```python
from build123d import *

# Parameters (mm, degrees)
SKETCH1_R           = 8.89
BOSS_EXTRUDE2_DEPTH = 9.525
SKETCH1_7_R         = 8.89
BOSS_EXTRUDE4_DEPTH = 22.225


with BuildPart() as part:
    # Sketch1 → Boss-Extrude2 (new body)
    # profile 1 of 5: a face of its own
    with BuildSketch(Plane(origin=(0, 0, 0), x_dir=(0, 0, -1), z_dir=(1, 0, 0))):
        with BuildLine():
            add(Edge.make_bspline(
                [(14.974900338, 11.775179823), (12.331090746, 14.230118369), (9.525, 16.497783942)],
                knots=[1.475431476, 1.475431476, 1.475431476, 1.652003752, 1.652003752, 1.652003752], degree=2, weights=[0.938489801, 0.965564284, 1]))
            ThreePointArc((9.525, 16.497783942), (4.930502809, 18.400886991), (0, 19.05))
            ThreePointArc((0, 19.05), (-10.677275343, 15.776510744), (-17.68505503, 7.0810542))
            add(Edge.make_bspline(
                [(-17.68505503, 7.0810542), (-18.489189379, 3.563978658), (-19.05, 0)],
                knots=[4.617024129, 4.617024129, 4.617024129, 4.793596405, 4.793596405, 4.793596405], degree=2, weights=[0.938489801, 0.965564284, 1]))
            ThreePointArc((-19.05, 0), (-18.400886991, -4.930502809), (-16.497783942, -9.525))
            ThreePointArc((-16.497783942, -9.525), (-8.324221416, -17.135047062), (2.710154692, -18.856234023))
            add(Edge.make_bspline(
                [(2.710154692, -18.856234023), (6.158098634, -17.794097027), (9.525, -16.497783942)],
                knots=[1.475431476, 1.475431476, 1.475431476, 1.652003752, 1.652003752, 1.652003752], degree=2, weights=[0.938489801, 0.965564284, 1]))
            ThreePointArc((9.525, -16.497783942), (13.470384182, -13.470384182), (16.497783942, -9.525))
            ThreePointArc((16.497783942, -9.525), (18.400886991, -4.930502809), (19.05, 0))
            ThreePointArc((19.05, 0), (18.002421385, 6.230194562), (14.974900338, 11.775179823))
        make_face()
        Circle(SKETCH1_R, mode=Mode.SUBTRACT)
    # profile 2 of 5: a face of its own
    with BuildSketch(Plane(origin=(0, 0, 0), x_dir=(0, 0, -1), z_dir=(1, 0, 0))):
        Circle(SKETCH1_R)
        Polygon((2.822954141, -4.8895), (5.645908282, 0), (2.822954141, 4.8895), (-2.822954141, 4.8895), (-5.645908282, 0), (-2.822954141, -4.8895), align=None, mode=Mode.SUBTRACT)
    # profile 3 of 5: a face of its own
    with BuildSketch(Plane(origin=(0, 0, 0), x_dir=(0, 0, -1), z_dir=(1, 0, 0))):
        with BuildLine():
            ThreePointArc((-17.68505503, 7.0810542), (-10.677275343, 15.776510744), (0, 19.05))
            ThreePointArc((0, 19.05), (2.161493982, 32.047813076), (8.413309173, 43.646520237))
            add(Edge.make_bspline(
                [(8.413309173, 43.646520237), (-8.576070469, 46.921395365), (-17.68505503, 7.0810542)],
                knots=[3.141592654, 3.141592654, 3.141592654, 4.617024129, 4.617024129, 4.617024129], degree=2, weights=[1, 0.712256416, 0.938489801]))
        make_face()
    # profile 4 of 5: a face of its own
    with BuildSketch(Plane(origin=(0, 0, 0), x_dir=(0, 0, -1), z_dir=(1, 0, 0))):
        with BuildLine():
            ThreePointArc((-16.497783942, -9.525), (-28.83496725, -14.151997839), (-42.005649898, -14.537120645))
            add(Edge.make_bspline(
                [(-42.005649898, -14.537120645), (-36.347085133, -30.887792574), (2.710154692, -18.856234023)],
                knots=[0, 0, 0, 1.475431476, 1.475431476, 1.475431476], degree=2, weights=[1, 0.712256416, 0.938489801]))
            ThreePointArc((2.710154692, -18.856234023), (-8.324221416, -17.135047062), (-16.497783942, -9.525))
        make_face()
    # profile 5 of 5: a face of its own
    with BuildSketch(Plane(origin=(0, 0, 0), x_dir=(0, 0, -1), z_dir=(1, 0, 0))):
        with BuildLine():
            add(Edge.make_bspline(
                [(33.592340725, -29.109399592), (44.923155602, -16.033602792), (14.974900338, 11.775179823)],
                knots=[0, 0, 0, 1.475431476, 1.475431476, 1.475431476], degree=2, weights=[1, 0.712256416, 0.938489801]))
            ThreePointArc((14.974900338, 11.775179823), (18.002421385, 6.230194562), (19.05, 0))
            ThreePointArc((19.05, 0), (18.400886991, -4.930502809), (16.497783942, -9.525))
            ThreePointArc((16.497783942, -9.525), (26.673473268, -17.895815237), (33.592340725, -29.109399592))
        make_face()
    extrude(amount=BOSS_EXTRUDE2_DEPTH)

    # Sketch1_7 → Boss-Extrude4 (add)
    with BuildSketch(Plane(origin=(0, 0, 0), x_dir=(0, 0, -1), z_dir=(1, 0, 0))):
        Circle(SKETCH1_7_R)
        Polygon((2.822954141, -4.8895), (5.645908282, 0), (2.822954141, 4.8895), (-2.822954141, 4.8895), (-5.645908282, 0), (-2.822954141, -4.8895), align=None, mode=Mode.SUBTRACT)
    extrude(amount=BOSS_EXTRUDE4_DEPTH)


solid = part.part
```
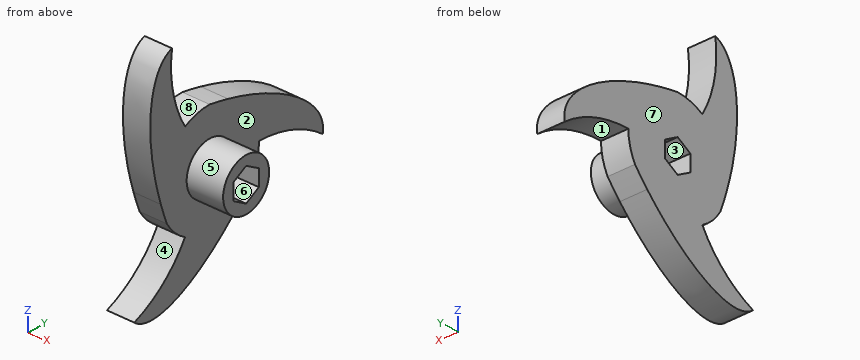
Verification items for the finished model (mm, model axes). Face numbers are marked on the shaded views. A direction names the side the tool comes from. Give positions to 0.01 mm unless a question says otherwise; leave off trailing zeros. Order: outer loops, then holes, each group sorted by start corner. A loop starts at its lowest first (then second) coordinate and runs counter-clockwise, first axis right, second up. Notation, with made-up numbers: M 79.25,54 L 120.25,54 A18 cw 120.25,64 Z; hole C 35,-21.75 d2. An arc over 180 degrees is marked long. Answer in a Markdown table with one row per item. Add a question column.
Item 1: Mould release check, pull along Y, two halves, no side actions. Record for the marked faces 5, 6, 7 and 8: released by +Y, released by -Y, zero draft, split by the parting line, or undercut.
Item 2: Tool access check on the marked faces 1, 2, 3 and 4. Record the directions out of +Z, -Z, +X, -X, +Y, -Y that give a thin tool (end or side, any length) a straight path to the whole face; none if there is none.
Item 3: Gauge pin test, flat ends, axial feed: pin 1 (1.7 mm diameter, centred on x = 6, z = -1, fed in from +Y); pin 2 (5 mm diameter, centred on x = 19, y = -3, fed in from -Z); pin 3 (4 mm diameter, centred on x = 5.5, y = -6.5, fed in from -Z); pin 4 (4 mm diameter, centred on x = 16, y = 12.5, fed in from +Z). Record the tip position at first contact, or that the pin passes through.
Item 4: Scan lines: probe 1 along X at (y, z) = (-5, -28) (3 decimals); probe 2 along Z at (x, y) = (19.5, 2); probe 3 along Z at (x, y) = (14, -1). Record each from-to range of solid material in increasing order. Write a range as from..to.
Item 5: Section check B-B, the plane z = -1. State how many separate pieces and enclosed holes the cut face has, and give its area (3 significant figures).
Item 6: Section check A-A, the plane x = 11.25. Enter the section's corners in (y, z).
Filled sheet:
| question | item | result |
|---|---|---|
| 1 | face 5 | split by the parting line |
| 1 | face 6 | undercut |
| 1 | face 7 | zero draft |
| 1 | face 8 | undercut |
| 2 | face 1 | -Z, +X, -X |
| 2 | face 2 | +X |
| 2 | face 3 | +X, -X |
| 2 | face 4 | +X, -X, -Y |
| 3 | pin 1 | stops at y = 42.37 |
| 3 | pin 2 | stops at z = -8.88 |
| 3 | pin 3 | stops at z = -31.37 |
| 3 | pin 4 | passes through |
| 4 | probe 1 | x = 0..9.525 |
| 4 | probe 2 | z = -8.66..-4.49, 4.49..8.66 |
| 4 | probe 3 | z = -8.83..-5.07, 5.07..8.83 |
| 5 | separate pieces | 3 |
| 5 | enclosed holes | 0 |
| 5 | area | 505 mm^2 |
| 6 | outline | C 0,0 d17.78; hole M -4.89,-2.82 L 0,-5.65 L 4.89,-2.82 L 4.89,2.82 L 0,5.65 L -4.89,2.82 Z |
